Check sheet for the drawn part. Datum: minimum x, y, z corner. Units: mm. A direction names the side the tool comes from. Round coordinates to 2 decimals unless told otherwise and drop trailing zeros. Write each loop counter-clockwise with the first axis right and the second up, starting at its lowest first coordinate (ties: lowest second). Pieces come first, ordered by that corner, then holes. Notation, with made-up numbers: (6.25, 22) - (27.25, 22) arc R18 cw to (27.25, 38) - close; hole circle Ø10 at (11.5, -18). An arc over 180 degrees is marked (long way). Answer as a JSON object with one key per item and string values. Group by question number.
1) Section check D-D (z = 34.5). Enter the section's corners in (x, y), then the cut area to 3 significant figures.
2) Section check A-A (x = 57.15). Enter the section's corners in (y, z), then the cut area to 3 significant figures.
3) Section check B-B (z = 19.05). Enter the section's corners in (x, y).
4) Mould release check, pull along X, two halves, no side actions. Record for the marked faces 4 and 5: +X half, -X half, draft (parallel to the pull), parting line (faces both ways), or undercut.
5) Thickness scan on line 1 (X direction, y = 74.4, z = 19.05); line 2 (Y direction, x = 7.5, z = 17); line 3 (Z direction, x = 19, y = 74). Record the ranges inside material, lowest first.
6) Set-up check for the marked faces 1, 2 and 3: record each of +Z, -Z, +X, -X, +Y, -Y from which the full face is reachable in a straight line by a thin tool's end or side.
7) Section check C-C (y = 67). Enter the section's corners in (x, z).
8) Go/stop test with flat-tipped pins: pin 1 Ø5 at (y, z) = (21, 26) entering from +X; pin 2 Ø11 at (x, y) = (12.5, 55.5) entering from +Z. Record where each tip stops, or that it passes through.
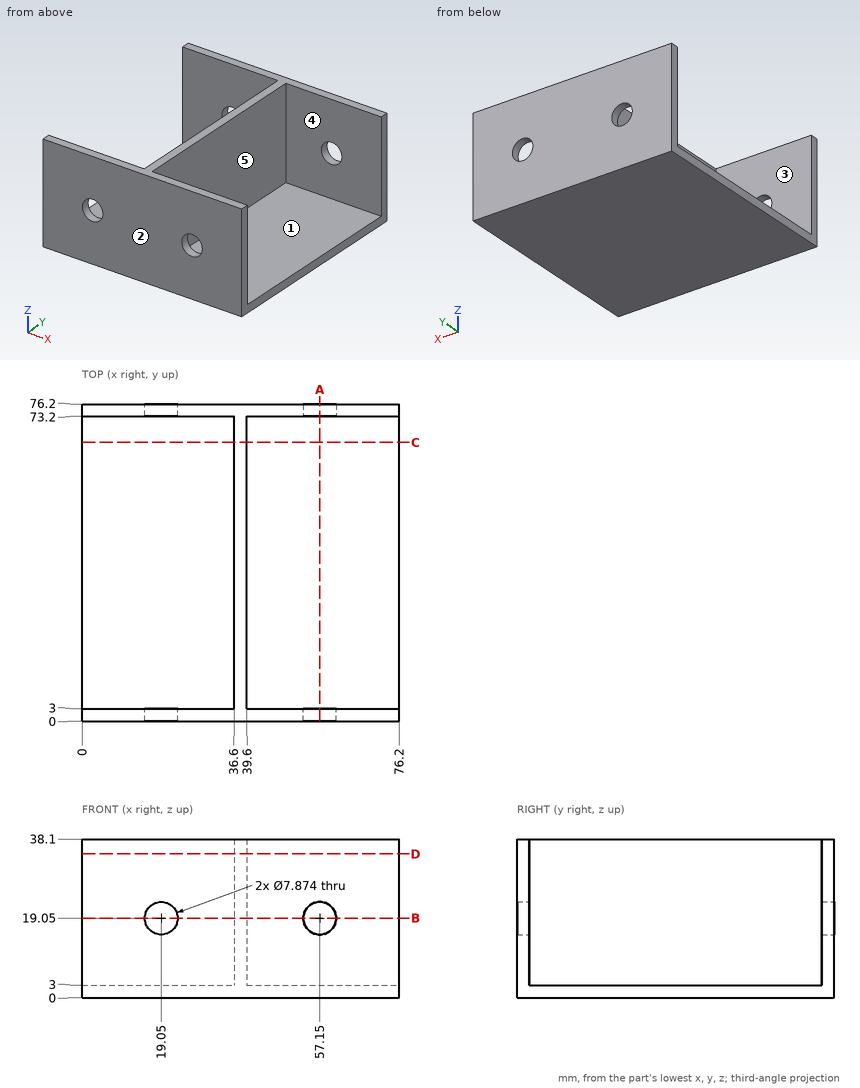
Returned:
{
 "1": {"outline": "(0, 0) - (76.2, 0) - (76.2, 3) - (39.6, 3) - (39.6, 73.2) - (76.2, 73.2) - (76.2, 76.2) - (0, 76.2) - (0, 73.2) - (36.6, 73.2) - (36.6, 3) - (0, 3) - close", "area": "668 mm2"},
 "2": {"outline": "(0, 0) - (76.2, 0) - (76.2, 15.11) - (73.2, 15.11) - (73.2, 3) - (3, 3) - (3, 15.11) - (0, 15.11) - close; (0, 22.99) - (3, 22.99) - (3, 38.1) - (0, 38.1) - close; (73.2, 22.99) - (76.2, 22.99) - (76.2, 38.1) - (73.2, 38.1) - close", "area": "392 mm2"},
 "3": {"outline": "(0, 0) - (15.11, 0) - (15.11, 3) - (0, 3) - close; (0, 73.2) - (15.11, 73.2) - (15.11, 76.2) - (0, 76.2) - close; (22.99, 0) - (53.21, 0) - (53.21, 3) - (39.6, 3) - (39.6, 73.2) - (53.21, 73.2) - (53.21, 76.2) - (22.99, 76.2) - (22.99, 73.2) - (36.6, 73.2) - (36.6, 3) - (22.99, 3) - close; (61.09, 0) - (76.2, 0) - (76.2, 3) - (61.09, 3) - close; (61.09, 73.2) - (76.2, 73.2) - (76.2, 76.2) - (61.09, 76.2) - close"},
 "4": {"face 4": "draft", "face 5": "+X half"},
 "5": {"line 1": "0 to 15.11, 22.99 to 53.21, 61.09 to 76.2", "line 2": "0 to 3, 73.2 to 76.2", "line 3": "0 to 15.11, 22.99 to 38.1"},
 "6": {"face 1": "+Z, +X", "face 2": "+Z, -Z, +X, -X, -Y", "face 3": "+Z, -X"},
 "7": {"outline": "(0, 0) - (76.2, 0) - (76.2, 3) - (39.6, 3) - (39.6, 38.1) - (36.6, 38.1) - (36.6, 3) - (0, 3) - close"},
 "8": {"pin 1": "x = 39.6", "pin 2": "z = 3"}
}
